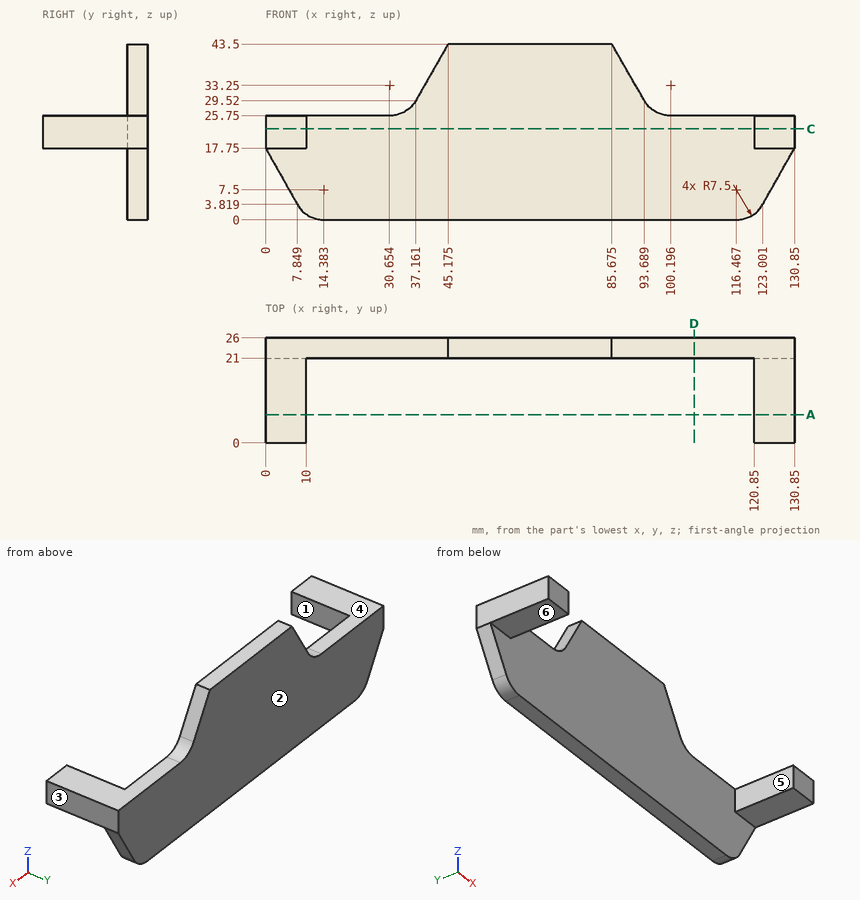
Here's the drawing with two shaded views (mm, measured from the low corner). I have some questions. A direction names the side the tool comes from. Coordinates: 2 decimals unless noted, no trailing zeros. Loops run counter-clockwise (first coordinate to the right, second up) from the corner with the lowest first, then second, coordinate; pieces in that order, holes last. Notation, with made-up numbers: M 47.5,-13.5 L 53.5,-13.5 A27 ccw 53.5,11.5 Z; hole C -23,65.25 d4. An arc over 180 degrees is marked long. Answer as CSV lines item,"result". Start each with the question number.
1. If I drill on probe 1 along Y at (x, z) = (28.5, 24.5); probe 2 along Z at (x, y) = (124, 10.75); probe 3 along X at (y, z) = (21.25, 16) (1 decimal), over which ranges is the centre line in solid material (lowest first)? Write a range as [from, to].
2. Suppose I cut it at C-C, the plane z = 22.5. List the corners of the cut face in (x, y) for me.
3. Thinking about a two-plate mould opening in X: for the marked faces 1, 2 and 3, which applies, +X half, -X half, draft (parallel to the pull), parting line (faces both ways), or undercut?
4. For the marked faces 4, 5 and 6, which set-ups out of +Z, -Z, +X, -X, +Y, -Y let a thin tool reach every point of the face, with its end or its side?
5. Suppose I cut it at A-A, the plane y = 7. List the corners of the cut face in (x, z) for me.
6. Suppose I cut it at D-D, the plane x = 106. List the corners of the cut face in (y, z) for me, plus the area to 3 significant figures.
7. For pin 1 Ø2 at (x, z) = (31.5, 26.5) entering from +Y; pin 2 Ø13 at (x, z) = (51, 15.5) entering from -Y; pin 3 Ø3 at (x, y) = (124, 15) entering from -Z; pin 4 Ø10 at (y, z) = (19.5, 35.5) entering from -X (1 decimal), each with a flat end and sliding along its axis, tell me the tip position at first contact or that it passes through.
Output:
1,probe 1,"y = [21, 26]"
1,probe 2,"z = [17.75, 25.75]"
1,probe 3,"x = [1, 129.9]"
2,outline,"M 0,0 L 10,0 L 10,21 L 120.85,21 L 120.85,0 L 130.85,0 L 130.85,26 L 0,26 Z"
3,face 1,"undercut"
3,face 2,"draft"
3,face 3,"+X half"
4,face 4,"+Z, -X, +Y, -Y"
4,face 5,"+Z, -Z, -Y"
4,face 6,"-Z, +X, -X, -Y"
5,outline,"M 0,17.75 L 10,17.75 L 10,25.75 L 0,25.75 Z; M 120.85,17.75 L 130.85,17.75 L 130.85,25.75 L 120.85,25.75 Z"
6,outline,"M 21,0 L 26,0 L 26,25.75 L 21,25.75 Z"
6,area,"129 mm^2"
7,pin 1,"stops at y = 26"
7,pin 2,"stops at y = 21"
7,pin 3,"stops at z = 17.75"
7,pin 4,"stops at x = 37.9"
